The model under review builds one solid part; all positions refer to its coordinate system, in mm. Face numbers are marked on the shaded views. Round coordinates to 2 decimals unless told otherwise and drop trailing zeros. Order: outer loops, then holes, each group sorted by start corner. A loop starts at its lowest first (then second) coordinate and runs counter-clockwise, first axis right, second up. Notation, with made-up numbers: M -38.75,-28.75 L 2.25,-28.75 A22 ccw 2.25,-6.75 Z; hole C -7,82.5 d8. An arc over 180 degrees is marked long. Use a Markdown table: item, result. Add a question column.
1. To check wall thickness, follow probe 1 along X at (y, z) = (104, 0); probe 2 along Y at (x, z) = (-14.65, 0); probe 3 along Z at (x, y) = (0.5, 178). State the ranges of each line that lie inside material, in increasing order.
2. Consider section A-A on x = 9. State the section outline as (y, z) points, then the cut area to 3 significant figures.
3. The part is to be moulded in two halves that separate along X. For the marked faces 1 and 2, say which applies: +X half, -X half, draft (parallel to the pull), parting line (faces both ways), or undercut.
4. Consider section C-C on y = 58. State the section outline as (x, z) points, then the cut area to 3 significant figures.
5. Insertion check: P1, Ø1, axis at y = 122.5, z = 5.5, coming from the -X side; P2, Ø2.5, axis at x = 0, y = 30, coming from the -Z side; P3, Ø12, axis at y = 132.5, z = 7.5, coming from the -X side; P4, Ø5, axis at y = 113, z = -7, coming from the +X side. Each pin has a flat end and moves straight along its axis. Give the tip position at first contact, or say it passes through.
6. Consider section B-B on z = 9. State the section outline as (x, y) points, then the cut area to 3 significant figures.
from build123d import *

# Parameters (mm, degrees)
SKETCH_1_R               = 15
EXTRUDE_1_DEPTH          = 273
CUT_EXTRUDE_1_DEPTH      = 274.822935489
CUT_EXTRUDE_1_DEPTH_BACK = 274.822935489
SKETCH_2_R               = 1.5
CUT_EXTRUDE_2_DEPTH      = 274.8229356
CUT_EXTRUDE_2_DEPTH_BACK = 274.8229356
SKETCH_3_R               = 1.5
CUT_EXTRUDE_3_REACH      = 275.823
SKETCH_4_R               = 14


with BuildPart() as part:
    # 草圖1 → 填料-伸長1 (new body)
    with BuildSketch(Plane(origin=(0, 0, 0), x_dir=(1, 0, 0), z_dir=(0, 1, 0))):
        with Locations(Location((0, 0, 0), (0, 0, 270))):
            Circle(SKETCH_1_R)
    extrude(amount=EXTRUDE_1_DEPTH)

    # 草圖2 → 除料-伸長1 (cut, two sides: drawn at the far end of the back side and taken through both)
    with BuildSketch(Plane.XY.offset(-CUT_EXTRUDE_1_DEPTH_BACK)):
        with Locations((0, 10)):
            Circle(SKETCH_2_R)
        with Locations((0, 30)):
            Circle(SKETCH_2_R)
        with Locations((0, 132)):
            Circle(SKETCH_2_R)
        with Locations((0, 152)):
            Circle(SKETCH_2_R)
    extrude(amount=CUT_EXTRUDE_1_DEPTH + CUT_EXTRUDE_1_DEPTH_BACK, mode=Mode.SUBTRACT)

    # 草圖3 → 除料-伸長2 (cut, two sides: drawn at the far end of the back side and taken through both)
    with BuildSketch(Plane(origin=(0, 0, 0), x_dir=(0, 0, -1), z_dir=(1, 0, 0)).offset(-CUT_EXTRUDE_2_DEPTH_BACK)):
        with Locations((0, 263)):
            Circle(SKETCH_3_R)
        with Locations((0, 243)):
            Circle(SKETCH_3_R)
    extrude(amount=CUT_EXTRUDE_2_DEPTH + CUT_EXTRUDE_2_DEPTH_BACK, mode=Mode.SUBTRACT)

    # 草圖4 → 除料-伸長3 (cut, up to next)
    with BuildSketch(Plane(origin=(0, 273, 0), x_dir=(1, 0, 0), z_dir=(0, 1, 0)), mode=Mode.PRIVATE) as cut_extrude_3_sk1:
        with Locations(Location((0, 0, 0), (0, 0, 270))):
            Circle(SKETCH_4_R)
    cut_extrude_3_tool1 = extrude(cut_extrude_3_sk1.sketch, amount=-CUT_EXTRUDE_3_REACH, mode=Mode.PRIVATE) & part.part
    add(cut_extrude_3_tool1.solids().sort_by_distance((0, 273, 0))[0], mode=Mode.SUBTRACT)


solid = part.part
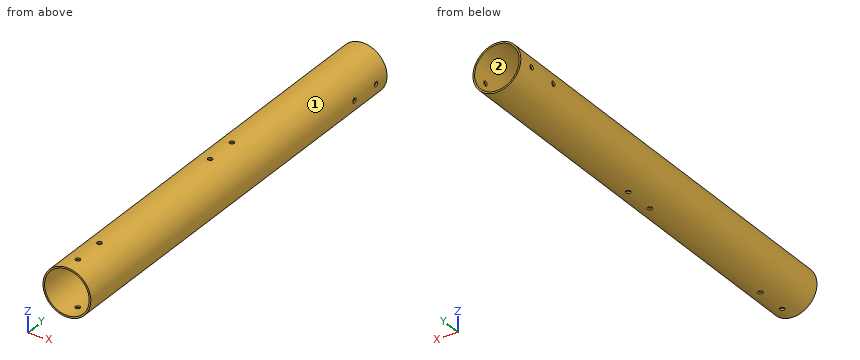
Answer block:
| question | item | result |
|---|---|---|
| 1 | probe 1 | -15 to -14, 14 to 15 |
| 1 | probe 2 | 0 to 241.5, 244.5 to 261.5, 264.5 to 273 |
| 1 | probe 3 | -14.99 to -13.99, 13.99 to 14.99 |
| 2 | outline | M 0,-12 L 273,-12 L 273,-10.72 L 0,-10.72 Z; M 0,10.72 L 273,10.72 L 273,12 L 0,12 Z |
| 2 | area | 697 mm^2 |
| 3 | face 1 | parting line |
| 3 | face 2 | undercut |
| 4 | outline | C 0,0 d30; hole C 0,0 d28 |
| 4 | area | 91.1 mm^2 |
| 5 | P1 | x = -14.14 |
| 5 | P2 | through |
| 5 | P3 | x = -14.92 |
| 5 | P4 | x = 14.31 |
| 6 | outline | M -12,0 L -10.72,0 L -10.72,273 L -12,273 Z; M 10.72,0 L 12,0 L 12,273 L 10.72,273 Z |
| 6 | area | 697 mm^2 |
